Autodesk Inventor part; units mm, degrees
ref_plane "YZ Plane" through (0, 0, 0) normal (1, 0, 0) x (0, 1, 0)
ref_plane "XZ Plane" through (0, 0, 0) normal (0, 1, 0) x (-1, 0, 0)
ref_plane "XY Plane" through (0, 0, 0) normal (0, 0, 1) x (1, 0, 0)
sketch "Sketch1" plane through (0, 0, 0) normal (0, 0, 1) x (1, 0, 0)
  circle A0 centre (0, 0) radius 2
  dimension "d0" = 4
extrude "Extrusion1" add sketch "Sketch1" along normal mid plane 16
fillet "Fillet1" radius 1 1 edges at (-2, 0, -8)
chamfer "Chamfer1" distance 0.5 angle 45 1 edges at (-2, 0, 8)
properties part number "DOWEL,M4X16" material "Steel"
Can you work these out from the model? Positions are in its coordinate system, mm. Coordinates: 2 decimals unless noted, no trailing zeros. Loops run counter-clockwise (first coordinate to the right, second up) from the corner with the lowest first, then second, coordinate; pieces in that order, holes last. Notation, with made-up numbers: M -13.75,-25.5 L -4.75,-25.5 A8 cw -4.75,-19.5 Z; hole C -37.75,18.25 d4. An arc over 180 degrees is marked long. Return JSON: item names as keys, results as strings. Group by question number.
Item 1: Imagine slicing it at A-A (z = -0.25). Please give me the cut outline in (x, y).
Item 2: If I drill on L1, parallel to Z at x = -1.05, y = -0.05; L2, parallel to Z at x = -0.75, y = -1.5; L3, parallel to X at y = 0.6, z = -4.75, over which ranges is the centre line in solid material (lowest first)? Write a range as from..to.
Item 3: I'm going to push a flat-ended pin straight in: pin 1 Ø1 at (x, y) = (1.5, 1) entering from -Z. Where does the tip first touch, or does it pass through?
Verdict:
{
 "1": {"outline": "C 0,0 d4"},
 "2": {"L1": "z = -8..8", "L2": "z = -7.74..7.82", "L3": "x = -1.91..1.91"},
 "3": {"pin 1": "stops at z = -7.95"}
}
